Autodesk Fusion 360 part; units mm, degrees
sketch "Schizzo1" plane through (0, 0, 0) normal (0, 1, 0) x (1, 0, 0)
  line L0 (0, 0) -> (-64.7048, -241.4815)
  line L1 (-64.7048, -241.4815) -> (-55.0455, -244.0696)
  line L2 (-55.0455, -244.0696) -> (4.9938, -20)
  line L3 (4.9938, -20) -> (250, -20)
  line L4 (250, -20) -> (250, 0)
  line L5 (250, 0) -> (0, 0)
  dimension "d1" = 75
  dimension "d2" = 250
  dimension "d3" = 250
  dimension "d4" = 20
  dimension "d5" = 10
extrude "Estrusione1" add sketch "Schizzo1" along normal blind 350
component "Component" placed x (1, 0, 0) y (0, 1, 0) z (0, 0, 1) at (0, 0, 0)
Check sheet for the modelled part. Datum: model origin and axes. Units: mm. A direction names the side the tool comes from. Round coordinates to 2 decimals unless told otherwise and drop trailing zeros. Loops run counter-clockwise (first coordinate to the right, second up) from the corner with the lowest first, then second, coordinate; pieces in that order, holes last. Notation, with made-up numbers: (18.5, -10) - (62.5, -10) arc R30 cw to (62.5, 14) - close; hole circle Ø2 at (19.25, 59). An arc over 180 degrees is marked (long way). Answer as a JSON object with one key per item and string values. Group by question number.
Q1. Sectioned sample at A-A, the plane y = 243. Enter the section's corners in (x, z).
Q2. Set-up check for faces 1 (the face through (127, 173, 0)), 2 (the face through (126, 173, 20)): record each of +Z, -Z, +X, -X, +Y, -Y from which the full face is reachable in a straight line by a thin tool's end or side.
Q3. Gauge pin test, flat ends, axial feed: P1, Ø6, axis at x = 10, y = 90.5, coming from the +Z side; P2, Ø1.5, axis at y = 83.5, z = 62.5, coming from the +X side; P3, Ø12, axis at y = 198, z = 40.5, coming from the +X side. Record the tip position at first contact, or that the pin passes through.
Q4. Sectioned sample at C-C, the plane z = 160.5. Enter the section's corners in (x, y).
Q5. Scan lines: line 1 along Z through (x, y) = (81.5, 25.5); line 2 along X through (y, z) = (84.5, 189); line 3 along X through (y, z) = (81, 146.5). Record each from-to range of solid material in increasing order. Write a range as [from, to].
Q6. Sectioned sample at B-B, the plane x = 94. Enter the section's corners in (y, z), plus the area to 3 significant figures.
Solution:
{
 "1": {"outline": "(-64.7, 241.48) - (0, 0) - (250, 0) - (250, 20) - (4.99, 20) - (-55.05, 244.07) - close"},
 "2": {"face 1": "-Z, +X, -X, +Y, -Y", "face 2": "+Z, +X, +Y, -Y"},
 "3": {"P1": "stops at z = 20", "P2": "stops at x = -6.19", "P3": "stops at x = 1.11"},
 "4": {"outline": "(-43.01, 0) - (-32.65, 0) - (-32.65, 350) - (-43.01, 350) - close"},
 "5": {"line 1": "z = [0, 20]", "line 2": "x = [-50.64, -40.29]", "line 3": "x = [-39.25, -28.9]"},
 "6": {"outline": "(0, 0) - (350, 0) - (350, 20) - (0, 20) - close", "area": "7,000 mm²"}
}
